from build123d import *

# Parameters (mm, degrees)
F0_R     = 45
F0_R_2   = 40
F1_DEPTH = 50
F0_R_3   = 50
F2_DEPTH = 100
F3_DEPTH = 5
F4_R     = 10


with BuildPart() as f1:
    # F0 (on Top) → F1 (new body)
    with BuildSketch(Plane.XY):
        Circle(F0_R)
        Circle(F0_R_2, mode=Mode.SUBTRACT)
    extrude(amount=F1_DEPTH)

    # F0 (on Top) → F2 (join)
    with BuildSketch(Plane.XY):
        Circle(F0_R_3)
        Circle(F0_R, mode=Mode.SUBTRACT)
    extrude(amount=F2_DEPTH)

    # F0 (on Top) → F3 (join)
    with BuildSketch(Plane.XY):
        Circle(F0_R_3)
        Circle(F0_R, mode=Mode.SUBTRACT)
        Circle(F0_R)
        Circle(F0_R_2, mode=Mode.SUBTRACT)
        Circle(F0_R_2)
    extrude(amount=F3_DEPTH)

    # F4
    f4_edges = [f1.edges().sort_by_distance(p)[0] for p in [
        (-50, 0, 0),
    ]]
    fillet(f4_edges, radius=F4_R)


solid = f1.part
Design review of the part built by this model. Coordinates are the model's own, in mm. A direction names the side the tool comes from. Round coordinates to 2 decimals unless told otherwise and drop trailing zeros. Write each loop counter-clockwise with the first axis right and the second up, starting at its lowest first coordinate (ties: lowest second). Pieces come first, ordered by that corner, then holes. Notation, with made-up numbers: (-2, 13) -> (5, 13) arc R17 ccw to (5, 35) -> close; hole circle Ø4 at (63, 70.5). An arc over 180 degrees is marked (long way). One line per item, written item: value. Start each with the question number.
Q1. Insertion check: P1, Ø4, axis at y = -7, z = 80, coming from the -X side; P2, Ø3, axis at x = -15.5, z = 76.5, coming from the +Y side; P3, Ø3, axis at y = -2, z = 55.5, coming from the -X side; P4, Ø1, axis at x = 33.5, y = 16, coming from the -Z side. Each pin has a flat end and moves straight along its axis. Give the tip position at first contact, or say it passes through.
Q2. Tool access review of faces 4 (the face through (-30.2, -26.5, 50)), 5 (the face through (-41, 19, 100)): name each direction out of +Z, -Z, +X, -X, +Y, -Y from which nothing blocks a thin tool from reaching the whole face with its end or side.
Q3. Add section C-C (z = 56). Give the boundary of the cut face in (x, y), then the cut area to 3 significant figures.
Q4. To check wall thickness, follow probe 1 along Y at (x, z) = (0, 18); probe 2 along Z at (x, y) = (30, 8.5); probe 3 along X at (y, z) = (-40, 86.5). State the ranges of each line that lie inside material, in increasing order.
Q5. Add section D-D (z = 26.5). Give the boundary of the cut face in (x, y).
Q6. Add section A-A (x = 0). Give the boundary of the cut face in (y, z).
Q7. The part is to be moulded in two halves that separate along Y. For faces 1 (the face through (47.69, 15.02, 54.37)), 2 (the face through (20.765, -39.923, 74.65)), 3 (the face through (-1, 1, 0)), say which applies: pulls with the +Y half, pulls with the -Y half, needs draft (parallel to the pull), parting line crosses it, or undercut.
Response:
1. P1: stops at x = -49.75
1. P2: stops at y = 48
1. P3: stops at x = -50
1. P4: stops at z = 0
2. face 4: +Z
2. face 5: +Z, +X, -X, +Y, -Y
3. outline: circle Ø100 at (0, 0); hole circle Ø90 at (0, 0)
3. area: 1,490 mm^2
4. probe 1: y = -50 to -40, 40 to 50
4. probe 2: z = 0 to 5
4. probe 3: x = -30 to -20.62, 20.62 to 30
5. outline: circle Ø100 at (0, 0); hole circle Ø80 at (0, 0)
6. outline: (-50, 10) arc R10 ccw to (-40, 0) -> (40, 0) arc R10 ccw to (50, 10) -> (50, 100) -> (45, 100) -> (45, 50) -> (40, 50) -> (40, 5) -> (-40, 5) -> (-40, 50) -> (-45, 50) -> (-45, 100) -> (-50, 100) -> close
7. face 1: parting line crosses it
7. face 2: undercut
7. face 3: needs draft
